```python
from build123d import *

# Parameters (mm, degrees)
SKETCH1_W                                            = 50
SKETCH1_H                                            = 125
BOSS_EXTRUDE1_DEPTH                                  = 5
SKETCH2_W                                            = 25
SKETCH2_H                                            = 93
CUT_EXTRUDE1_DEPTH                                   = 69.053287944
SKETCH3_W                                            = 10
SKETCH3_H                                            = 50
CUT_EXTRUDE2_DEPTH                                   = 69.053287944
CUT_EXTRUDE3_DEPTH                                   = 2
M4_TAPPED_HOLE1_D                                    = 3.3
SKETCH7_W                                            = 15
SKETCH7_H                                            = 25
CUT_EXTRUDE4_DEPTH                                   = 69.053287944
CBORE_FOR_M4_SLOTTED_CHEESE_HEAD_SCREWS2_D           = 4.5
CBORE_FOR_M4_SLOTTED_CHEESE_HEAD_SCREWS2_CBORE_D     = 8
CBORE_FOR_M4_SLOTTED_CHEESE_HEAD_SCREWS2_CBORE_DEPTH = 4.6
CBORE_FOR_M4_SLOTTED_CHEESE_HEAD_SCREWS3_D           = 4.5
CBORE_FOR_M4_SLOTTED_CHEESE_HEAD_SCREWS3_CBORE_D     = 8
CBORE_FOR_M4_SLOTTED_CHEESE_HEAD_SCREWS3_CBORE_DEPTH = 4.6
CHAMFER1_SIZE                                        = 10
FILLET1_R                                            = 5
FILLET2_R                                            = 2
CHAMFER2_SIZE                                        = 3
FILLET3_R                                            = 3
CHAMFER3_SIZE                                        = 1


# Some blends are built 0.0001 mm under size
with BuildPart() as part:
    # Sketch1 → Boss-Extrude1 (new, symmetric)
    with BuildSketch(Plane.XY):
        Rectangle(SKETCH1_W, SKETCH1_H)
    extrude(amount=BOSS_EXTRUDE1_DEPTH, both=True)

    # Sketch2 → Cut-Extrude1 (cut, through all)
    with BuildSketch(Plane.XY.offset(5)):
        with Locations((-12.5, 0)):
            Rectangle(SKETCH2_W, SKETCH2_H)
    extrude(amount=-CUT_EXTRUDE1_DEPTH, mode=Mode.SUBTRACT)

    # Sketch3 → Cut-Extrude2 (cut, through all)
    with BuildSketch(Plane.XY.offset(5)):
        with Locations((20, 0)):
            Rectangle(SKETCH3_W, SKETCH3_H)
    extrude(amount=-CUT_EXTRUDE2_DEPTH, mode=Mode.SUBTRACT)

    # Sketch4 → Cut-Extrude3 (cut)
    with BuildSketch(Plane(origin=(0, 0, -5), x_dir=(-1, 0, 0), z_dir=(0, 0, -1))):
        with BuildLine():
            Line((9.5, -57.5), (12.763932023, -57.5))
            ThreePointArc((12.763932023, -57.5), (12, -55.5), (12.763932023, -53.5))
            Line((12.763932023, -53.5), (9.5, -53.5))
            ThreePointArc((9.5, -53.5), (7.5, -55.5), (9.5, -57.5))
        make_face()
        with BuildLine():
            Line((12.763932023, -57.5), (17.236067977, -57.5))
            ThreePointArc((17.236067977, -57.5), (17.802517077, -56.570466269), (18, -55.5))
            ThreePointArc((18, -55.5), (17.802517077, -54.429533731), (17.236067977, -53.5))
            Line((17.236067977, -53.5), (12.763932023, -53.5))
            ThreePointArc((12.763932023, -53.5), (12, -55.5), (12.763932023, -57.5))
        make_face()
        with BuildLine():
            Line((12.763932023, -53.5), (17.236067977, -53.5))
            ThreePointArc((17.236067977, -53.5), (15, -52.5), (12.763932023, -53.5))
        make_face()
        with BuildLine():
            Line((17.236067977, -57.5), (20.5, -57.5))
            ThreePointArc((20.5, -57.5), (22.5, -55.5), (20.5, -53.5))
            Line((20.5, -53.5), (17.236067977, -53.5))
            ThreePointArc((17.236067977, -53.5), (17.802517077, -54.429533731), (18, -55.5))
            ThreePointArc((18, -55.5), (17.802517077, -56.570466269), (17.236067977, -57.5))
        make_face()
        with BuildLine():
            ThreePointArc((12.763932023, -57.5), (15, -58.5), (17.236067977, -57.5))
            Line((17.236067977, -57.5), (12.763932023, -57.5))
        make_face()
        with BuildLine():
            ThreePointArc((12.763932023, 53.5), (12, 55.5), (12.763932023, 57.5))
            Line((12.763932023, 57.5), (9.5, 57.5))
            ThreePointArc((9.5, 57.5), (7.5, 55.5), (9.5, 53.5))
            Line((9.5, 53.5), (12.763932023, 53.5))
        make_face()
        with BuildLine():
            Line((12.763932023, 57.5), (17.236067977, 57.5))
            ThreePointArc((17.236067977, 57.5), (15, 58.5), (12.763932023, 57.5))
        make_face()
        with BuildLine():
            ThreePointArc((18, 55.5), (17.802517077, 56.570466269), (17.236067977, 57.5))
            Line((17.236067977, 57.5), (12.763932023, 57.5))
            ThreePointArc((12.763932023, 57.5), (12, 55.5), (12.763932023, 53.5))
            Line((12.763932023, 53.5), (17.236067977, 53.5))
            ThreePointArc((17.236067977, 53.5), (17.802517077, 54.429533731), (18, 55.5))
        make_face()
        with BuildLine():
            ThreePointArc((20.5, 53.5), (22.5, 55.5), (20.5, 57.5))
            Line((20.5, 57.5), (17.236067977, 57.5))
            ThreePointArc((17.236067977, 57.5), (17.802517077, 56.570466269), (18, 55.5))
            ThreePointArc((18, 55.5), (17.802517077, 54.429533731), (17.236067977, 53.5))
            Line((17.236067977, 53.5), (20.5, 53.5))
        make_face()
        with BuildLine():
            ThreePointArc((12.763932023, 53.5), (15, 52.5), (17.236067977, 53.5))
            Line((17.236067977, 53.5), (12.763932023, 53.5))
        make_face()
    extrude(amount=-CUT_EXTRUDE3_DEPTH, mode=Mode.SUBTRACT)

    # M4 Tapped Hole1 (through all)
    with Locations(Plane(origin=(0, 0, -5), x_dir=(-1, 0, 0), z_dir=(0, 0, -1))):
        with Locations((15, -55.5), (15, 55.5)):
            Hole(M4_TAPPED_HOLE1_D / 2)

    # Sketch7 → Cut-Extrude4 (cut, through all)
    with BuildSketch(Plane(origin=(0, 0, -5), x_dir=(-1, 0, 0), z_dir=(0, 0, -1))):
        with Locations((-17.5, -50)):
            Rectangle(SKETCH7_W, SKETCH7_H)
        with Locations((-17.5, 50)):
            Rectangle(SKETCH7_W, SKETCH7_H)
    extrude(amount=-CUT_EXTRUDE4_DEPTH, mode=Mode.SUBTRACT)

    # CBORE for M4 Slotted cheese head screws2 (through all)
    with Locations(Plane(origin=(0, -37.5, 0), x_dir=(-1, 0, 0), z_dir=(0, -1, 0))):
        with Locations((-20, 0)):
            cbore_for_m4_slotted_cheese_head_screws2 = CounterBoreHole(CBORE_FOR_M4_SLOTTED_CHEESE_HEAD_SCREWS2_D / 2, CBORE_FOR_M4_SLOTTED_CHEESE_HEAD_SCREWS2_CBORE_D / 2, CBORE_FOR_M4_SLOTTED_CHEESE_HEAD_SCREWS2_CBORE_DEPTH)

    # CBORE for M4 Slotted cheese head screws3 (through all)
    with Locations(Plane.ZY):
        with Locations((0, 0)):
            CounterBoreHole(CBORE_FOR_M4_SLOTTED_CHEESE_HEAD_SCREWS3_D / 2, CBORE_FOR_M4_SLOTTED_CHEESE_HEAD_SCREWS3_CBORE_D / 2, CBORE_FOR_M4_SLOTTED_CHEESE_HEAD_SCREWS3_CBORE_DEPTH)

    # Mirror1: CBORE for M4 Slotted cheese head screws2 across plane
    add(cbore_for_m4_slotted_cheese_head_screws2.mirror(Plane.ZX), mode=Mode.SUBTRACT)

    # Chamfer1
    # the kernel refuses this chamfer: 10 mm, written as the material it adds along each edge
    with BuildSketch(Plane(origin=(10, -37.5, -5), x_dir=(-0.027495876610586317, -0.9996219169112968, 0), z_dir=(0, 0, 1))) as chamfer1_piece_1_section:
        Polygon((CHAMFER1_SIZE * 0.999621916911, CHAMFER1_SIZE * 0.0274958766106), (-CHAMFER1_SIZE * 0.0274958766106, CHAMFER1_SIZE * 0.999621916911), (0, 0), align=None)
    chamfer1_piece_1 = extrude(amount=10, mode=Mode.PRIVATE)
    chamfer1_piece_1 = chamfer1_piece_1 - Plane(origin=(20, -41.045650517, 0), x_dir=(-1, 0, 0), z_dir=(0, -1, 0)) * Cylinder(4, 60, mode=Mode.PRIVATE)
    add(chamfer1_piece_1)
    with BuildSketch(Plane(origin=(10, 37.5, -5), x_dir=(-0.027495876610586317, 0.9996219169112968, 0), z_dir=(0, 0, 1))) as chamfer1_piece_2_section:
        Polygon((CHAMFER1_SIZE * 0.999621916911, -CHAMFER1_SIZE * 0.0274958766106), (-CHAMFER1_SIZE * 0.0274958766106, -CHAMFER1_SIZE * 0.999621916911), (0, 0), align=None)
    chamfer1_piece_2 = extrude(amount=10, mode=Mode.PRIVATE)
    chamfer1_piece_2 = chamfer1_piece_2 - Plane(origin=(20, 41.045650517, 0), x_dir=(-1, 0, 0), z_dir=(0, 1, 0)) * Cylinder(4, 60, mode=Mode.PRIVATE)
    add(chamfer1_piece_2)

    # Fillet1
    # the kernel refuses this fillet: 5 mm, written as the material it adds along each edge
    with BuildSketch(Plane(origin=(10, -47.5, -5), x_dir=(0.707106781186831, 0.707106781186264, 0), z_dir=(0, 0, 1))) as fillet1_piece_1:
        with BuildLine():
            CenterArc((FILLET1_R * 0.414213562373, -FILLET1_R), FILLET1_R, 90, 45)
            Line((-FILLET1_R * 0.292893218814, -FILLET1_R * 0.292893218814), (0, 0))
            Line((0, 0), (FILLET1_R * 0.414213562373, 0))
        make_face()
    extrude(amount=10)
    with BuildSketch(Plane(origin=(20, -37.5, -5), x_dir=(-0.7071067811868298, -0.7071067811862654, 0), z_dir=(0, 0, 1))) as fillet1_piece_2_section:
        with BuildLine():
            CenterArc((FILLET1_R * 0.414213562373, FILLET1_R), FILLET1_R, 225, 45)
            Line((-FILLET1_R * 0.292893218813, FILLET1_R * 0.292893218813), (0, 0))
            Line((0, 0), (FILLET1_R * 0.414213562373, 0))
        make_face()
    fillet1_piece_2 = extrude(amount=6.17766953, mode=Mode.PRIVATE)
    fillet1_piece_2 = fillet1_piece_2 - Plane(origin=(20, -37.809724496, 0), x_dir=(-1, 0, 0), z_dir=(0, -1, 0)) * Cylinder(4, 21, mode=Mode.PRIVATE)
    add(fillet1_piece_2)
    with BuildSketch(Plane(origin=(10, 47.5, -5), x_dir=(0.707106781186831, -0.707106781186264, 0), z_dir=(0, 0, 1))) as fillet1_piece_3:
        with BuildLine():
            CenterArc((FILLET1_R * 0.414213562373, FILLET1_R), FILLET1_R, 225, 45)
            Line((-FILLET1_R * 0.292893218814, FILLET1_R * 0.292893218814), (0, 0))
            Line((0, 0), (FILLET1_R * 0.414213562373, 0))
        make_face()
    extrude(amount=10)
    with BuildSketch(Plane(origin=(20, 37.5, -5), x_dir=(-0.7071067811868298, 0.7071067811862654, 0), z_dir=(0, 0, 1))) as fillet1_piece_4_section:
        with BuildLine():
            CenterArc((FILLET1_R * 0.414213562373, -FILLET1_R), FILLET1_R, 90, 45)
            Line((-FILLET1_R * 0.292893218813, -FILLET1_R * 0.292893218813), (0, 0))
            Line((0, 0), (FILLET1_R * 0.414213562373, 0))
        make_face()
    fillet1_piece_4 = extrude(amount=6.17766953, mode=Mode.PRIVATE)
    fillet1_piece_4 = fillet1_piece_4 - Plane(origin=(20, 37.8097245, 0), x_dir=(-1, 0, 0), z_dir=(0, 1, 0)) * Cylinder(4, 21, mode=Mode.PRIVATE)
    add(fillet1_piece_4)
    with BuildSketch(Plane(origin=(20, -37.5, -1.17766953), x_dir=(-0.7071067811868306, -0.7071067811862645, 0), z_dir=(0, 0, 1))) as fillet1_piece_5_section:
        with BuildLine():
            CenterArc((FILLET1_R * 0.414213562373, FILLET1_R), FILLET1_R, 225, 45)
            Line((-FILLET1_R * 0.292893218813, FILLET1_R * 0.292893218813), (0, 0))
            Line((0, 0), (FILLET1_R * 0.414213562373, 0))
        make_face()
    fillet1_piece_5 = extrude(amount=6.17766953, mode=Mode.PRIVATE)
    fillet1_piece_5 = fillet1_piece_5 - Plane(origin=(20, -37.8097245, 0), x_dir=(-1, 0, 0), z_dir=(0, -1, 0)) * Cylinder(4, 21, mode=Mode.PRIVATE)
    add(fillet1_piece_5)
    with BuildSketch(Plane(origin=(20, 37.5, -1.17766953), x_dir=(-0.7071067811868306, 0.7071067811862645, 0), z_dir=(0, 0, 1))) as fillet1_piece_6_section:
        with BuildLine():
            CenterArc((FILLET1_R * 0.414213562373, -FILLET1_R), FILLET1_R, 90, 45)
            Line((-FILLET1_R * 0.292893218813, -FILLET1_R * 0.292893218813), (0, 0))
            Line((0, 0), (FILLET1_R * 0.414213562373, 0))
        make_face()
    fillet1_piece_6 = extrude(amount=6.17766953, mode=Mode.PRIVATE)
    fillet1_piece_6 = fillet1_piece_6 - Plane(origin=(20, 37.809724496, 0), x_dir=(-1, 0, 0), z_dir=(0, 1, 0)) * Cylinder(4, 21, mode=Mode.PRIVATE)
    add(fillet1_piece_6)

    # Fillet2
    fillet2_edges = [part.edges().sort_by_distance(p)[0] for p in [
        (0, 46.5, 0),
        (0, -46.5, 0),
        (15, -25, 0),
        (15, 25, 0),
    ]]
    fillet(fillet2_edges, radius=FILLET2_R)

    # Chamfer2
    chamfer2_edges = [part.edges().sort_by_distance(p)[0] for p in [
        (10, -62.5, 0),
        (10, 62.5, 0),
        (-25, 62.5, 0),
        (-25, -62.5, 0),
    ]]
    chamfer(chamfer2_edges, length=CHAMFER2_SIZE)

    # Fillet3
    fillet3_edges = [part.edges().sort_by_distance(p)[0] for p in [
        (7, -62.5, 0),
        (7, 62.5, 0),
        (10, -59.5, 0),
        (10, 59.5, 0),
    ]]
    fillet(fillet3_edges, radius=FILLET3_R)

    # Chamfer3
    chamfer3_edges = [part.edges().sort_by_distance(p)[0] for p in [
        (23.535533906, 37.5, 5),
        (-25, -53, 5),
        (15, -42.5, 5),
        (23.535533906, -37.5, 5),
        (10, 53.914213562, 5),
        (15, 42.5, 5),
        (10.380602337, -47.65765065, 5),
        (20.15765065, -37.880602337, 5),
        (10.380602337, 47.65765065, 5),
        (20.15765065, 37.880602337, 5),
        (15, 0, 5),
        (21, -25, 5),
        (15.585786438, 24.414213562, 5),
        (15.585786438, -24.414213562, 5),
        (-8.121320344, -62.5, 5),
        (-8.121320344, 62.5, 5),
        (-25, 53, 5),
        (-23.5, 61, 5),
        (-23.5, -61, 5),
        (8.5, 61, 5),
        (8.5, -61, 5),
        (10, -53.914213562, 5),
        (6.90540961, -62.271638598, 5),
        (9.771638598, -59.40540961, 5),
        (9.771638598, 59.40540961, 5),
        (6.90540961, 62.271638598, 5),
        (21, 25, 5),
    ]]
    chamfer(chamfer3_edges, length=CHAMFER3_SIZE - 0.0001)  # a hair under: the kernel refuses the full size


solid = part.part
```
The listing builds one solid part. Answer for the finished solid, in the listing's coordinates (mm). A direction names the side the tool comes from. Coordinates: 2 decimals unless noted, no trailing zeros. Write each loop counter-clockwise with the first axis right and the second up, starting at its lowest first coordinate (ties: lowest second). Pieces come first, ordered by that corner, then holes.
Q1. Section C-C, the plane y = -31.5 is taken. Write down the section's boundary in (x, z), then the cut area to 3 significant figures.
Returned:
outline: (0, -5) - (25, -5) - (25, 5) - (0, 5) - close; hole circle Ø4.5 at (20, 0)
area: 234 mm2
Q2. Section A-A, the plane x = -15 is taken. Write down the section's boundary in (y, z), then the cut area to 3 significant figures.
Returned:
outline: (-62.5, -5) - (-58.5, -5) - (-58.5, -3) - (-57.15, -3) - (-57.15, 5) - (-61.5, 5) - (-62.5, 4) - close; (-53.85, -3) - (-52.5, -3) - (-52.5, -5) - (-46.5, -5) - (-46.5, 5) - (-53.85, 5) - close; (46.5, -5) - (52.5, -5) - (52.5, -3) - (53.85, -3) - (53.85, 5) - (46.5, 5) - close; (57.15, -3) - (58.5, -3) - (58.5, -5) - (62.5, -5) - (62.5, 4) - (61.5, 5) - (57.15, 5) - close
area: 242 mm2
Q3. The mould has two halves that part along Z. Classify faces 1 (the cylindrical face through (16.29, -36.3, -1.49)), 2 (the cylindrical face through (-13.476, 54.868, 1.056)), 3 (the flat face through (3, 0, 5)): released by +Z, released by -Z, zero draft, split by the parting line, or undercut.
Returned:
face 1: undercut
face 2: zero draft
face 3: released by +Z
Q4. Section B-B, the plane y = -55.5 is taken. Write down the section's boundary in (x, z).
Returned:
outline: (-25, -5) - (-22.5, -5) - (-22.5, -3) - (-16.65, -3) - (-16.65, 5) - (-24, 5) - (-25, 4) - close; (-13.35, -3) - (-7.5, -3) - (-7.5, -5) - (10, -5) - (10, 4) - (9, 5) - (-13.35, 5) - close
Q5. Find the intervals of material crossed by line 1 along Y through (x, z) = (-15, 1.5); line 2 along Z through (x, y) = (20, 28.5); line 3 along Y through (x, z) = (4, -0.25), in increasing order.
Returned:
line 1: y = -62.5 to -57.15, -53.85 to -46.5, 46.5 to 53.85, 57.15 to 62.5
line 2: z = -5 to -2.25, 2.25 to 5
line 3: y = -62.5 to -3.99, 3.99 to 62.5
Q6. Given P1, Ø3.5, axis at x = 20, z = 0, coming from the +Y side; P2, Ø3, axis at x = 9.5, z = 0, coming from the -Y side; P3, Ø1.5, axis at y = 28.5, z = 1.5, coming from the -X side; P4, Ø3, axis at y = -0.5, z = 1, coming from the -X side, each flat-ended and moving along its own axis, determine where each tip first touches the part or whether it passes through.
Returned:
P1: passes through
P2: stops at y = -61.5
P3: stops at x = 0
P4: stops at x = 4.6
Q7. Which of the six approach directions +Z, -Z, +X, -X, +Y, -Y give full straight-line access (tool end or side, diameter ignored) to faces 4 (the flat face through (0, -0.6, -4.4)), 5 (the flat face through (10, -54, -1)), 6 (the flat face through (10, 54, -1)), 7 (the flat face through (14.602, 42.201, 4.493)), 8 (the flat face through (-13, 56, -3))?
Returned:
face 4: +Z, -Z, -X
face 5: +Z, -Z, +X, -Y
face 6: +Z, -Z, +X, +Y
face 7: +Z, +X, +Y
face 8: -Z
